```python
from build123d import *

# Parameters (mm, degrees)
SKETCH1_R           = 5
BOSS_EXTRUDE1_DEPTH = 30
SKETCH2_R           = 2
CUT_EXTRUDE1_DEPTH  = 31
SKETCH4_R           = 15
SKETCH4_R_2         = 5
BOSS_EXTRUDE3_DEPTH = 3


with BuildPart() as part:
    # Sketch1 → Boss-Extrude1 (new body)
    with BuildSketch(Plane.XY):
        Circle(SKETCH1_R)
    extrude(amount=BOSS_EXTRUDE1_DEPTH)

    # Sketch2 → Cut-Extrude1 (cut, through all)
    with BuildSketch(Plane.XY.offset(30)):
        Circle(SKETCH2_R)
    extrude(amount=-CUT_EXTRUDE1_DEPTH, mode=Mode.SUBTRACT)

    # Sketch4 → Boss-Extrude3 (add)
    with BuildSketch(Plane.XY.offset(30)):
        Circle(SKETCH4_R)
        Circle(SKETCH4_R_2, mode=Mode.SUBTRACT)
    extrude(amount=-BOSS_EXTRUDE3_DEPTH)


solid = part.part
```
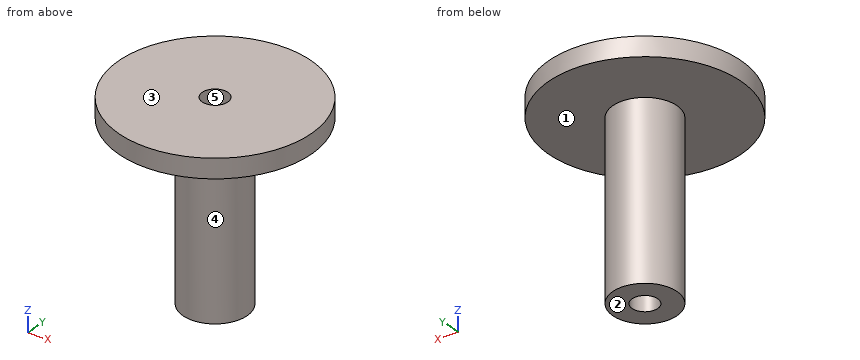
Check sheet for the modelled part. Datum: model origin and axes. Units: mm. Face numbers are marked on the shaded views. A direction names the side the tool comes from. Give positions to 0.01 mm unless a question says otherwise; leave off trailing zeros. Loops run counter-clockwise (first coordinate to the right, second up) from the corner with the lowest first, then second, coordinate; pieces in that order, holes last. Notation, with made-up numbers: (-8, -34) - (14, -34) arc R17 ccw to (14, -1) - close; hole circle Ø2 at (77, 78.5). An arc over 180 degrees is marked (long way). One line per question, with ' | ' between items. Start each with the question number.
1. Cross-section at A-A, the plane y = 0. Enter the section's corners in (x, z).
2. Gauge pin test, flat ends, axial feed: pin 1 Ø6 at (x, y) = (-11, -10) entering from -Z; pin 2 Ø8 at (y, z) = (-3.5, 14) entering from -X; pin 3 Ø5 at (y, z) = (6.5, 22.5) entering from +X; pin 4 Ø3.5 at (x, y) = (0, 0) entering from -Z. Record the tip position at first contact, or that the pin passes through.
3. Material ranges on line 1 along Y through (x, z) = (0, 11.25); line 2 along Z through (x, y) = (-3.5, -13.5); line 3 along Y through (x, z) = (1.25, 12), recorded low to high. Write a range as [from, to].
4. Cross-section at C-C, the plane z = 8. Enter the section's corners in (x, y), plus the area to 3 significant figures.
5. Cross-section at D-D, the plane y = 12. Enter the section's corners in (x, z).
6. Draft check along Y on the marked faces 3, 4 and 5. Enter one of: released by +Y, released by -Y, zero draft, split by the parting line, or undercut.
7. Set-up check for the marked faces 1 and 2: record each of +Z, -Z, +X, -X, +Y, -Y from which the full face is reachable in a straight line by a thin tool's end or side.
Check result:
1) outline: (-15, 27) - (-5, 27) - (-5, 0) - (-2, 0) - (-2, 30) - (-15, 30) - close; (2, 0) - (5, 0) - (5, 27) - (15, 27) - (15, 30) - (2, 30) - close
2) pin 1: stops at z = 27 | pin 2: stops at x = -5 | pin 3: stops at x = 3 | pin 4: passes through
3) line 1: y = [-5, -2], [2, 5] | line 2: z = [27, 30] | line 3: y = [-4.84, -1.56], [1.56, 4.84]
4) outline: circle Ø10 at (0, 0); hole circle Ø4 at (0, 0) | area: 66.0 mm2
5) outline: (-9, 27) - (9, 27) - (9, 30) - (-9, 30) - close
6) face 3: zero draft | face 4: split by the parting line | face 5: undercut
7) face 1: -Z | face 2: -Z, +X, -X, +Y, -Y
